Input: part model. Units: mm. Frame: model coordinates. Face numbers are marked on the shaded views. A direction names the side the tool comes from. Give positions to 0.01 mm unless a question says otherwise; leave off trailing zeros. Loops run counter-clockwise (first coordinate to the right, second up) from the corner with the lowest first, then second, coordinate; pieces in that order, holes last.
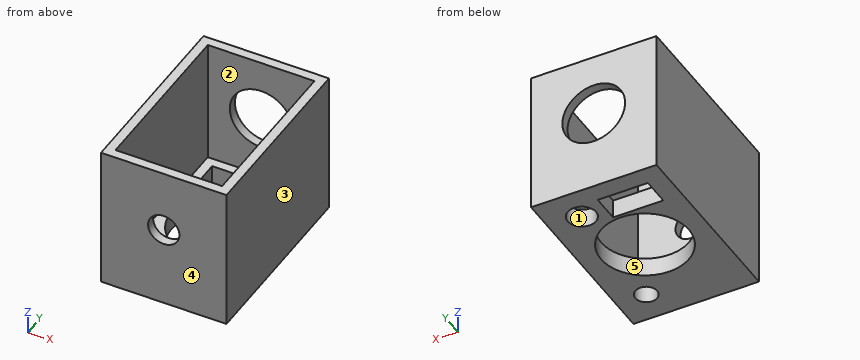
from build123d import *

# Parameters (mm, degrees)
SKETCH1_W           = 20
SKETCH1_H           = 30
SKETCH1_W_2         = 8
SKETCH1_H_2         = 4.5
SKETCH1_R           = 1.75
SKETCH1_R_2         = 2.25
SKETCH1_R_3         = 7
BOSS_EXTRUDE1_DEPTH = 3
SKETCH1_3_W         = 20
SKETCH1_3_H         = 30
SKETCH1_3_W_2       = 17
SKETCH1_3_H_2       = 27
BOSS_EXTRUDE2_DEPTH = 20
SKETCH2_R           = 2.5
CUT_EXTRUDE1_DEPTH  = 42.231056256
CUT_EXTRUDE2_START  = -28.5
SKETCH2_3_R         = 5
SKETCH2_3_R_2       = 2.5
CUT_EXTRUDE2_DEPTH  = 13.731056256


with BuildPart() as part:
    # Sketch1 → Boss-Extrude1 (new body)
    with BuildSketch(Plane.XY):
        with Locations((10, 35)):
            Rectangle(SKETCH1_W, SKETCH1_H)
        with Locations((7, 44.75)):
            Rectangle(SKETCH1_W_2, SKETCH1_H_2, mode=Mode.SUBTRACT)
        with Locations((15.25, 25)):
            Circle(SKETCH1_R, mode=Mode.SUBTRACT)
        with Locations((14.75, 44.75)):
            Circle(SKETCH1_R_2, mode=Mode.SUBTRACT)
        with Locations((10, 35)):
            Circle(SKETCH1_R_3, mode=Mode.SUBTRACT)
    extrude(amount=-BOSS_EXTRUDE1_DEPTH)

    # Sketch1<3> → Boss-Extrude2 (add)
    with BuildSketch(Plane.XY):
        with Locations((10, 35)):
            Rectangle(SKETCH1_3_W, SKETCH1_3_H)
        with Locations((10, 35)):
            Rectangle(SKETCH1_3_W_2, SKETCH1_3_H_2, mode=Mode.SUBTRACT)
    extrude(amount=BOSS_EXTRUDE2_DEPTH)

    # Sketch2 → Cut-Extrude1 (cut, through all)
    with BuildSketch(Plane.XZ.offset(-20)):
        with Locations((10, 10)):
            Circle(SKETCH2_R)
    extrude(amount=-CUT_EXTRUDE1_DEPTH, mode=Mode.SUBTRACT)

    # Sketch2<3> → Cut-Extrude2 (cut, through all)
    with BuildSketch(Plane.XZ.offset(-20).offset(CUT_EXTRUDE2_START)):
        with Locations((10, 10)):
            Circle(SKETCH2_3_R)
        with Locations((10, 10)):
            Circle(SKETCH2_3_R_2, mode=Mode.SUBTRACT)
    extrude(amount=-CUT_EXTRUDE2_DEPTH, mode=Mode.SUBTRACT)


solid = part.part
(1) Pin query (flat end, axial travel): pin 1 Ø5 at (x, y) = (8, 39.5) entering from +Z; pin 2 Ø8.5 at (x, y) = (10, 35) entering from +Z. Return the tip coordinate at first contact, or that it passes through.
Values follow:
pin 1: stops at z = 0
pin 2: passes through
(2) Cut plane A-A (x = 10). Return the cut outline in (y, z), and give its area (3 significant figures).
Values follow:
outline: (20, -3) - (28, -3) - (28, 0) - (21.5, 0) - (21.5, 7.5) - (20, 7.5) - close; (20, 12.5) - (21.5, 12.5) - (21.5, 20) - (20, 20) - close; (42, -3) - (42.5, -3) - (42.5, 0) - (42, 0) - close; (47, -3) - (50, -3) - (50, 5) - (48.5, 5) - (48.5, 0) - (47, 0) - close; (48.5, 15) - (50, 15) - (50, 20) - (48.5, 20) - close
area: 72.0 mm2
(3) Mould query, pull axis Y, two halves, no side actions, for the marked faces 3, 4 and 5. Classes: +Y half, -Y half, draft (parallel to the pull), parting line (faces both ways), or undercut.
Values follow:
face 3: draft
face 4: -Y half
face 5: undercut
(4) Reachability of the marked faces 1 and 2 from +Z, -Z, +X, -X, +Y, -Y: full face, straight path, thin tool, end or side. Return the list, or none.
Values follow:
face 1: +Z, -Z
face 2: +Z
(5) Cut plane D-D (x = 17.75). Return the cut outline in (y, z).
Values follow:
outline: (20, -3) - (50, -3) - (50, 20) - (48.5, 20) - (48.5, 0) - (21.5, 0) - (21.5, 20) - (20, 20) - close
(6) Cut plane B-B (y = 44.75). Return the cut outline in (x, z), and give its area (3 significant figures).
Values follow:
outline: (0, -3) - (3, -3) - (3, 0) - (1.5, 0) - (1.5, 20) - (0, 20) - close; (11, -3) - (12.5, -3) - (12.5, 0) - (11, 0) - close; (17, -3) - (20, -3) - (20, 20) - (18.5, 20) - (18.5, 0) - (17, 0) - close
area: 82.5 mm2
(7) Cut plane C-C (z = -1). Return the cut outline in (x, y).
Values follow:
outline: (0, 20) - (20, 20) - (20, 50) - (0, 50) - close; hole circle Ø14 at (10, 35); hole (3, 42.5) - (11, 42.5) - (11, 47) - (3, 47) - close; hole circle Ø4.5 at (14.75, 44.75); hole circle Ø3.5 at (15.25, 25)
(8) Ray query, probe 1 along Y at (x, z) = (10, -0.9); probe 2 along Y at (x, z) = (15.75, 2.5); probe 3 along Z at (x, y) = (10.25, 48.75). Return the intervals inside material, ascending.
Values follow:
probe 1: y = 20 to 28, 42 to 42.5, 47 to 50
probe 2: y = 20 to 21.5, 48.5 to 50
probe 3: z = -3 to 5.01, 14.99 to 20
